Check sheet for the modelled part. Datum: model origin and axes. Units: mm. A direction names the side the tool comes from. Give positions to 0.01 mm unless a question says otherwise; leave off trailing zeros. Write each loop counter-clockwise with the first axis right and the second up, starting at its lowest first coordinate (ties: lowest second). Pieces come first, ordered by that corner, then holes. Notation, with made-up numbers: M 16,84 L 59,84 A36 cw 59,120 Z; hole C 36.25,66.25 d1. An arc over 180 degrees is marked long. Write item = value, one per line. Start each with the question number.
1) Scan lines: L1, parallel to Z at x = 16, y = 0; L2, parallel to Z at x = -0.35, y = 0; L3, parallel to X at y = 10.5, z = -12. Record each from-to range of solid material in increasing order.
2) Gauge pin test, flat ends, axial feed: pin 1 (1.5 mm diameter, centred on x = -2.5, z = 10, fed in from +Y); pin 2 (6 mm diameter, centred on y = -14, z = 17.5, fed in from +X); pin 3 (5 mm diameter, centred on x = 19.5, z = 32, fed in from +Y). Record the tip position at first contact, or that the pin passes through.
3) Sectioned sample at C-C, the plane x = 18. Record the cut outline in (y, z).
4) Set-up check for faces 1 (the face through (-6.056, -7.91, -10.316)), 2 (the face through (-0.5, 0.8, -11.5)), 3 (the face through (-1.26, -10.74, -2.38)): record each of +Z, -Z, +X, -X, +Y, -Y from which the full face is reachable in a straight line by a thin tool's end or side.
5) Sectioned sample at A-A, the plane y = 0. Record the cut outline in (x, z).
from build123d import *

# Parameters (mm, degrees)
FILLET1_R          = 5
SKETCH3_R          = 11
CUT_EXTRUDE2_DEPTH = 41
SKETCH6_W          = 0.5
SKETCH6_H          = 55
SKETCH9_R          = 13
CUT_EXTRUDE3_DEPTH = 8


with BuildPart() as part:
    # Sketch1 → Revolve1 (revolve)
    with BuildSketch(Plane.XY):
        Polygon((0, 0), (0, 81), (30, 81), (30, 84), (-10, 84), (-10, 0), align=None)
    revolve(axis=Axis((-10, 0, 0), (1, 0, 0)))

    # Fillet1
    fillet1_edges = [part.edges().sort_by_distance(p)[0] for p in [
        (-10, -84, 0),
    ]]
    fillet(fillet1_edges, radius=FILLET1_R)

    # Sketch3 → Cut-Extrude2 (cut, through all)
    with BuildSketch(Plane.ZY.offset(10)):
        Circle(SKETCH3_R)
    extrude(amount=-CUT_EXTRUDE2_DEPTH, mode=Mode.SUBTRACT)

    # Sketch6 → Cut-Revolve2 (revolve, cut)
    with BuildSketch(Plane.XY):
        with Locations((-0.25, 27.5)):
            Rectangle(SKETCH6_W, SKETCH6_H)
    revolve(axis=Axis((-10, 0, 0), (1, 0, 0)), mode=Mode.SUBTRACT)

    # Sketch9 → Cut-Extrude3 (cut)
    with BuildSketch(Plane.ZY.offset(10)):
        Circle(SKETCH9_R)
    extrude(amount=-CUT_EXTRUDE3_DEPTH, mode=Mode.SUBTRACT)


solid = part.part
Data:
q1.L1 = -84 to -81, 81 to 84
q1.L2 = -84 to -55, 55 to 84
q1.L3 = -10 to -0.5
q2.pin_1 = 83.49
q2.pin_2 = -0.5
q2.pin_3 = 78.65
q3.outline = C 0,0 d168; hole C 0,0 d162
q4.face_1 = -X
q4.face_2 = +X
q4.face_3 = +X, -X
q5.outline = M -10,-79 A5 ccw -5,-84 L 30,-84 L 30,-81 L 0,-81 L 0,-55 L -0.5,-55 L -0.5,-11 L -2,-11 L -2,-13 L -10,-13 Z; M -10,13 L -2,13 L -2,11 L -0.5,11 L -0.5,55 L 0,55 L 0,81 L 30,81 L 30,84 L -5,84 A5 ccw -10,79 Z
